Geometry: final body of the model. Coordinates: model frame, mm. A direction names the side the tool comes from. Coordinates: 2 decimals unless noted, no trailing zeros. Write each loop counter-clockwise with the first axis right and the second up, starting at its lowest first coordinate (ties: lowest second). Pieces come first, ordered by that corner, then holes. Notation, with made-up numbers: (-4.5, 69) - (9.5, 69) arc R19 cw to (9.5, 73) - close; hole circle Ø2 at (79, 27.25). An arc over 180 degrees is marked (long way). Answer as a JSON object with one key per item and string values. Group by question number.
Item 1: Section A-A on z = 30.3. Return loops of the section in (x, y).
Item 2: Set-up query: faces 1 (the cylindrical face through (-2.58, 4.05, 1.49)), 2 (the flat face through (4, -4, 12)), 3 (the flat face through (0, 5, 35)), 4 (the flat face through (-0.1, -2.2, 0)). Return all of +Z, -Z, +X, -X, +Y, -Y with unobstructed straight access to the full face (end or side cutting, diameter ignored); none if empty.
Item 3: Section D-D on z = 9. Return loops of the section in (x, y), and give its area (3 significant figures).
Item 4: First-contact query: pin 1 Ø5 at (x, z) = (-5, 40.3) entering from -Y; pin 2 Ø5 at (x, y) = (1.5, 1) entering from +Z; pin 3 Ø1.8 at (x, z) = (-5, 30.3) entering from +Y; pin 4 Ø6 at (x, z) = (-2, 16) entering from +Y. Flat tips, straight axial feed; report the tip coordinate or a pass-through.
Item 5: Mould query, pull axis Y, two halves, no side actions, for faces 5 (the flat face through (-0.1, 2.3, 25.3)), 6 (the cylindrical face through (-1.08, -4.88, 6.93)), 7 (the flat face through (0, 8, 34)). Classes: pulls with the +Y half, pulls with the -Y half, needs draft (parallel to the pull), parting line crosses it, or undercut.
Item 6: Line query: line 1 along X through (y, z) = (-5.65, 30.3); line 2 along Y through (x, z) = (2.5, 32); line 3 along Z through (x, y) = (-2, 2.75). Output: solid intervals per line, ascending. Write a range as from..to.
Item 7: Section B-B on x = 0. Return loops of the section in (y, z).
Item 8: Section C-C on y = 6.5. Return loops of the section in (x, z), and give its area (3 significant figures).
```python
from build123d import *

# Parameters (mm, degrees)
SKETCH_1_R          = 5
EXTRUDE_1_DEPTH     = 12
SKETCH_2_R          = 5
SKETCH_2_R_2        = 4.8
CUT_EXTRUDE_1_DEPTH = 1
SKETCH_3_R          = 6
EXTRUDE_2_DEPTH     = 10.3
SKETCH_4_W          = 20
SKETCH_4_H          = 16
EXTRUDE_3_DEPTH     = 23
SKETCH_5_W          = 20
SKETCH_5_H          = 10
CUT_EXTRUDE_3_DEPTH = 20
SKETCH_6_R          = 1.5
CUT_EXTRUDE_4_DEPTH = 20
FILLET_1_R          = 5
SKETCH_7_R          = 2
CUT_EXTRUDE_5_DEPTH = 48.075365107


with BuildPart() as part:
    # 草图1 → 凸台-拉伸1 (new body)
    with BuildSketch(Plane.XY):
        Circle(SKETCH_1_R)
    extrude(amount=EXTRUDE_1_DEPTH)

    # 草图2 → 切除-拉伸1 (cut)
    with BuildSketch(Plane(origin=(0, 0, 1), x_dir=(-1, 0, 0), z_dir=(0, 0, -1))):
        Circle(SKETCH_2_R)
        Circle(SKETCH_2_R_2, mode=Mode.SUBTRACT)
    extrude(amount=-CUT_EXTRUDE_1_DEPTH, mode=Mode.SUBTRACT)

    # 草图3 → 凸台-拉伸2 (add)
    with BuildSketch(Plane.XY.offset(12)):
        with Locations(Location((0, 0, 0), (0, 0, 180))):
            Circle(SKETCH_3_R)
    extrude(amount=EXTRUDE_2_DEPTH)

    # 草图4 → 凸台-拉伸3 (add)
    with BuildSketch(Plane.XY.offset(22.3)):
        Rectangle(SKETCH_4_W, SKETCH_4_H)
    extrude(amount=EXTRUDE_3_DEPTH)

    # 草图5 → 切除-拉伸3 (cut)
    with BuildSketch(Plane.XY.offset(45.3)):
        Rectangle(SKETCH_5_W, SKETCH_5_H)
    extrude(amount=-CUT_EXTRUDE_3_DEPTH, mode=Mode.SUBTRACT)

    # 草图6 → 切除-拉伸4 (cut)
    with BuildSketch(Plane(origin=(0, 8, 0), x_dir=(1, 0, 0), z_dir=(0, 1, 0))):
        with Locations(Location((5, -40.3, 0), (0, 0, 270))):
            Circle(SKETCH_6_R)
        with Locations(Location((-5, -40.3, 0), (0, 0, 270))):
            Circle(SKETCH_6_R)
        with Locations(Location((-5, -30.3, 0), (0, 0, 270))):
            Circle(SKETCH_6_R)
        with Locations(Location((5, -30.3, 0), (0, 0, 270))):
            Circle(SKETCH_6_R)
    extrude(amount=-CUT_EXTRUDE_4_DEPTH, mode=Mode.SUBTRACT)

    # 圆角1
    fillet_1_edges = [part.edges().sort_by_distance(p)[0] for p in [
        (10, -6.5, 45.3),
        (-10, 6.5, 45.3),
        (10, 6.5, 45.3),
        (-10, -6.5, 45.3),
    ]]
    fillet(fillet_1_edges, radius=FILLET_1_R)

    # 草图7 → 切除-拉伸5 (cut, through all)
    with BuildSketch(Plane(origin=(0, 0, 0), x_dir=(-1, 0, 0), z_dir=(0, 0, -1))):
        Circle(SKETCH_7_R)
    extrude(amount=-CUT_EXTRUDE_5_DEPTH, mode=Mode.SUBTRACT)


solid = part.part
```
Checks:
{
 "1": {"outline": "(-10, -8) - (-6.5, -8) - (-6.5, -5) - (-10, -5) - close; (-10, 5) - (-6.5, 5) - (-6.5, 8) - (-10, 8) - close; (-3.5, -8) - (3.5, -8) - (3.5, -5) - (-3.5, -5) - close; (-3.5, 5) - (3.5, 5) - (3.5, 8) - (-3.5, 8) - close; (6.5, -8) - (10, -8) - (10, -5) - (6.5, -5) - close; (6.5, 5) - (10, 5) - (10, 8) - (6.5, 8) - close"},
 "2": {"face 1": "none", "face 2": "-Z", "face 3": "+Z, +X, -X", "face 4": "-Z, +X, -X, +Y, -Y"},
 "3": {"outline": "circle Ø10 at (0, 0); hole circle Ø4 at (0, 0)", "area": "66.0 mm^2"},
 "4": {"pin 1": "y = -8", "pin 2": "z = 25.3", "pin 3": "through", "pin 4": "y = 6"},
 "5": {"face 5": "undercut", "face 6": "parting line crosses it", "face 7": "pulls with the +Y half"},
 "6": {"line 1": "-10..-6.5, -3.5..3.5, 6.5..10", "line 2": "-8..-5, 5..8", "line 3": "0..25.3"},
 "7": {"outline": "(-8, 22.3) - (-6, 22.3) - (-6, 12) - (-5, 12) - (-5, 2) - (-4.8, 2) - (-4.8, 1) - (-5, 1) - (-5, 0) - (-2, 0) - (-2, 25.3) - (-5, 25.3) - (-5, 45.3) - (-8, 45.3) - close; (2, 0) - (5, 0) - (5, 1) - (4.8, 1) - (4.8, 2) - (5, 2) - (5, 12) - (6, 12) - (6, 22.3) - (8, 22.3) - (8, 45.3) - (5, 45.3) - (5, 25.3) - (2, 25.3) - close"},
 "8": {"outline": "(-10, 22.3) - (10, 22.3) - (10, 40.3) arc R5 ccw to (5, 45.3) - (-5, 45.3) arc R5 ccw to (-10, 40.3) - close; hole circle Ø3 at (-5, 30.3); hole circle Ø3 at (-5, 40.3); hole circle Ø3 at (5, 30.3); hole circle Ø3 at (5, 40.3)", "area": "421 mm^2"}
}
